Could you check a few things on this model? Use its own coordinates, in mm. Face numbers are marked on the shaded views. Coordinates: 2 decimals unless noted, no trailing zeros. Loops run counter-clockwise (first coordinate to the right, second up) from the corner with the lowest first, then second, coordinate; pieces in that order, holes last. Notation, with made-up numbers: (-12.5, 39.25) -> (-2.5, 39.25) arc R20 ccw to (-2.5, 72.25) -> close; hole circle Ø9 at (74, 45). An arc over 180 degrees is marked (long way). One line per question, with ' | ' between items. Start each with the question number.
(1) If I drill on line 1 along X through (y, z) = (4.5, 52.5); line 2 along X through (y, z) = (2, -4); line 3 along Z through (x, y) = (39.5, 1), over which ranges is the centre line in solid material (lowest first)?
(2) Suppose I cut it at A-A (x = -41). Please give me the cut outline in (y, z).
(3) Suppose I cut it at B-B (x = 101.5). Please give me the cut outline in (y, z), plus the area to 3 significant figures.
(4) Suppose I cut it at C-C (y = 9.75). Please give me the cut outline in (x, z).
(5) I'm going to push flat-ended pins straight in: pin 1 Ø3 at (x, z) = (88.5, 72) entering from -Y; pin 2 Ø0.5 at (y, z) = (6.5, 40.5) entering from +X; pin 3 Ø12 at (x, z) = (-4.5, 30.5) entering from +Y. Where does each tip first touch, or does it pass through?
(6) If we mould it in two halves opening along Z, with no side actions, what happens to the marked faces 1, 2 and 3? For each: pulls with the +Z half, pulls with the -Z half, needs draft (parallel to the pull), parting line crosses it, or undercut.
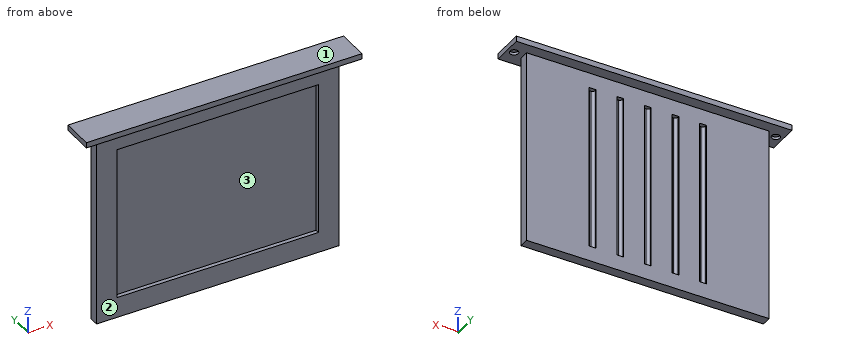
```python
from build123d import *

# Parameters (mm, degrees)
SKETCH1_W           = 176
SKETCH1_H           = 142
BOSS_EXTRUDE1_DEPTH = 7
SKETCH2_W           = 192
SKETCH2_H           = 23
BOSS_EXTRUDE2_DEPTH = 4
SKETCH3_W           = 146
SKETCH3_H           = 112
CUT_EXTRUDE1_DEPTH  = 3
SKETCH4_W           = 5
SKETCH4_H           = 120
CUT_EXTRUDE2_DEPTH  = 3
FILLET1_R           = 2
SKETCH6_W           = 4
SKETCH6_H           = 23
BOSS_EXTRUDE3_DEPTH = 4
SKETCH7_W           = 4
SKETCH7_H           = 23
BOSS_EXTRUDE4_DEPTH = 4
SKETCH5_R           = 3
CUT_EXTRUDE3_DEPTH  = 190.179668735
SKETCH8_R           = 3
BOSS_EXTRUDE5_DEPTH = 2


with BuildPart() as part:
    # Sketch1 → Boss-Extrude1 (new body)
    with BuildSketch(Plane(origin=(0, 0, 0), x_dir=(1, 0, 0), z_dir=(0, 1, 0))):
        with Locations((19.364764745, -37.446274738)):
            Rectangle(SKETCH1_W, SKETCH1_H)
    extrude(amount=BOSS_EXTRUDE1_DEPTH)

    # Sketch2 → Boss-Extrude2 (add)
    with BuildSketch(Plane.XY.offset(108.446274738)):
        with Locations((19.364764745, 3.5)):
            Rectangle(SKETCH2_W, SKETCH2_H)
    extrude(amount=BOSS_EXTRUDE2_DEPTH)

    # Sketch3 → Cut-Extrude1 (cut)
    with BuildSketch(Plane.XZ):
        with Locations((19.364764745, 37.446274738)):
            Rectangle(SKETCH3_W, SKETCH3_H)
    extrude(amount=-CUT_EXTRUDE1_DEPTH, mode=Mode.SUBTRACT)

    # Sketch4 → Cut-Extrude2 (cut)
    with BuildSketch(Plane(origin=(0, 7, 0), x_dir=(1, 0, 0), z_dir=(0, 1, 0))):
        with Locations((19.364764745, -37.446274738)):
            Rectangle(SKETCH4_W, SKETCH4_H)
        with Locations((39.364764745, -37.446274738)):
            Rectangle(SKETCH4_W, SKETCH4_H)
        with Locations((-0.635235255, -37.446274738)):
            Rectangle(SKETCH4_W, SKETCH4_H)
        with Locations((59.364764745, -37.446274738)):
            Rectangle(SKETCH4_W, SKETCH4_H)
        with Locations((-20.635235255, -37.446274738)):
            Rectangle(SKETCH4_W, SKETCH4_H)
    extrude(amount=-CUT_EXTRUDE2_DEPTH, mode=Mode.SUBTRACT)

    # Fillet1
    fillet1_edges = [part.edges().sort_by_distance(p)[0] for p in [
        (41.864764745, 4, 37.446274738),
        (36.864764745, 4, 37.446274738),
        (-3.135235255, 4, 37.446274738),
        (1.864764745, 4, 37.446274738),
        (61.864764745, 4, 37.446274738),
        (56.864764745, 4, 37.446274738),
        (-23.135235255, 4, 37.446274738),
        (-18.135235255, 4, 37.446274738),
        (21.864764745, 4, 37.446274738),
        (16.864764745, 4, 37.446274738),
    ]]
    fillet(fillet1_edges, radius=FILLET1_R)

    # Sketch6 → Boss-Extrude3 (add)
    with BuildSketch(Plane.ZY.offset(76.635235255)):
        with Locations((110.446274738, 3.5)):
            Rectangle(SKETCH6_W, SKETCH6_H)
    extrude(amount=BOSS_EXTRUDE3_DEPTH)

    # Sketch7 → Boss-Extrude4 (add)
    with BuildSketch(Plane(origin=(115.364764745, 0, 0), x_dir=(0, 0, -1), z_dir=(1, 0, 0))):
        with Locations((-110.446274738, 3.5)):
            Rectangle(SKETCH7_W, SKETCH7_H)
    extrude(amount=BOSS_EXTRUDE4_DEPTH)

    # Sketch5 → Cut-Extrude3 (cut, through all)
    with BuildSketch(Plane.XY.offset(112.446274738)):
        with Locations((-75.635235255, 3.5)):
            Circle(SKETCH5_R)
        with Locations((114.364764745, 3.5)):
            Circle(SKETCH5_R)
    extrude(amount=-CUT_EXTRUDE3_DEPTH, mode=Mode.SUBTRACT)

    # Sketch8 → Boss-Extrude5 (add)
    with BuildSketch(Plane.XY.offset(112.446274738)):
        with Locations((-75.635235255, 3.5)):
            Circle(SKETCH8_R)
        with Locations((114.364764745, 3.5)):
            Circle(SKETCH8_R)
    extrude(amount=-BOSS_EXTRUDE5_DEPTH)


solid = part.part
```
Checks:
1) line 1: x = -68.64 to -22.46, -18.81 to -2.46, 1.19 to 17.54, 21.19 to 37.54, 41.19 to 57.54, 61.19 to 107.36 | line 2: x = -68.64 to -53.64, 92.36 to 107.36 | line 3: z = -33.55 to -18.55, 93.45 to 112.45
2) outline: (-8, 108.45) -> (0, 108.45) -> (0, 93.45) -> (3, 93.45) -> (3, -18.55) -> (0, -18.55) -> (0, -33.55) -> (7, -33.55) -> (7, 108.45) -> (15, 108.45) -> (15, 112.45) -> (-8, 112.45) -> close
3) outline: (-8, 108.45) -> (0, 108.45) -> (0, -33.55) -> (7, -33.55) -> (7, 108.45) -> (15, 108.45) -> (15, 112.45) -> (-8, 112.45) -> close | area: 1,090 mm^2
4) outline: (-80.64, 108.45) -> (119.36, 108.45) -> (119.36, 112.45) -> (-80.64, 112.45) -> close
5) pin 1: stops at y = 3 | pin 2: stops at x = 107.36 | pin 3: stops at y = 7
6) face 1: pulls with the +Z half | face 2: needs draft | face 3: undercut
